Here's how the part is built. I have some questions about the finished solid (model axes, mm). Face numbers are marked on the shaded views. A direction names the side the tool comes from. Round coordinates to 2 decimals unless told otherwise and drop trailing zeros. Loops run counter-clockwise (first coordinate to the right, second up) from the corner with the lowest first, then second, coordinate; pieces in that order, holes last. Notation, with made-up numbers: (69.25, 65.25) - (90.25, 65.25) arc R8 ccw to (90.25, 71.25) - close; hole circle Ø7 at (32, -1.75). An arc over 180 degrees is marked (long way). Answer as a JSON object with one key per item and string values. Group by question number.
1) Will these pins go through, and if not, where does the flat tip stop? P1, Ø16.5, axis at y = -9, z = 69, coming from the -X side; P2, Ø16.5, axis at y = 9, z = 68.5, coming from the +X side; P3, Ø3, axis at x = 8, y = -3.5, coming from the -Z side; P4, Ø4.5, axis at x = 51.5, z = 33.23, coming from the +Y side.
2) I want a section at C-C, the plane x = 44.5. Please give me the cut outline in (y, z), then the cut area to 3 significant figures.
3) I want a section at D-D, the plane z = -2.5. Please give me the cut outline in (x, y), then the cut area to 3 significant figures.
4) I want a section at A-A, the plane z = -43. Please give me the cut outline in (x, y).
5) I want a section at B-B, the plane y = 16. Please give me the cut outline in (x, z).
6) Which directions (+Z, -Z, +X, -X, +Y, -Y) give clear straight access to the entire face, cutting with the end or side of a thin tool? Please do the marked faces 1, 2 and 3.
7) If I drill on line 1 along X through (y, z) = (1.5, -43); line 2 along Z through (x, y) = (-50, 14); line 3 along X through (y, z) = (-14, -9), over which ranges is the centre line in solid material (lowest first)? Write a range as [from, to].
from build123d import *

# Parameters (mm, degrees)
BASE_MODEL_DEPTH         = 19
F_5_0_5_DIAMETER_HOLE1_D = 5


with BuildPart() as part:
    # Top → Base Model (new, symmetric)
    with BuildSketch(Plane(origin=(0, 0, 0), x_dir=(1, 0, 0), z_dir=(0, 1, 0))):
        with BuildLine():
            Line((-5.390272104, 50.397653109), (-58.548817366, -28.484658378))
            ThreePointArc((-58.548817366, -28.484658378), (-59.931398216, -32.157094268), (-59.517033361, -36.059224064))
            Line((-59.517033361, -36.059224064), (-51, -60.234834557))
            Line((-51, -60.234834557), (-51, -75.234834557))
            Line((-51, -75.234834557), (51, -75.234834557))
            Line((51, -75.234834557), (51, -60.234834557))
            Line((51, -60.234834557), (59.517033361, -36.059224064))
            ThreePointArc((59.517033361, -36.059224064), (59.931398216, -32.157094268), (58.548817366, -28.484658378))
            Line((58.548817366, -28.484658378), (5.390272104, 50.397653109))
            ThreePointArc((5.390272104, 50.397653109), (3.052771705, 52.503683101), (0, 53.265165443))
            ThreePointArc((0, 53.265165443), (-3.052771705, 52.503683101), (-5.390272104, 50.397653109))
        make_face()
    extrude(amount=BASE_MODEL_DEPTH, both=True)

    # Ø5.0 (5) Diameter Hole1 (through all)
    with Locations(Plane(origin=(0, 19, 0), x_dir=(1, 0, 0), z_dir=(0, 1, 0))):
        with Locations((-51.5, -33.234834557), (0, 43), (51.5, -33.234834557)):
            Hole(F_5_0_5_DIAMETER_HOLE1_D / 2)


solid = part.part
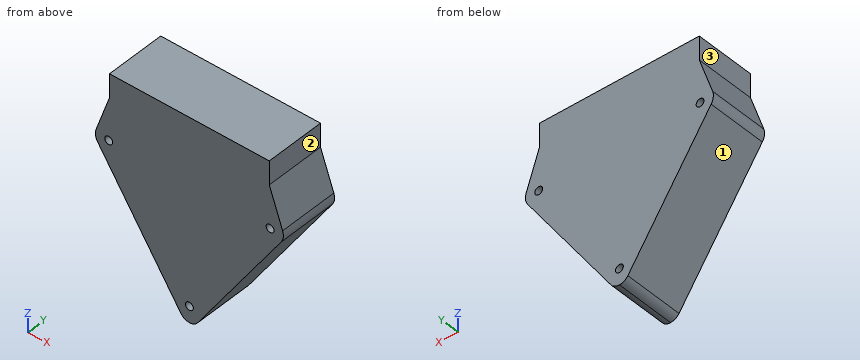
Outcome:
{
 "1": {"P1": "x = -51", "P2": "x = 51", "P3": "z = -48.75", "P4": "through"},
 "2": {"outline": "(-19, 7.64) - (19, 7.64) - (19, 75.23) - (-19, 75.23) - close", "area": "2,570 mm^2"},
 "3": {"outline": "(-37.67, -19) - (37.67, -19) - (37.67, 19) - (-37.67, 19) - close", "area": "2,860 mm^2"},
 "4": {"outline": "(-10.38, -19) - (-2.5, -19) - (-2.5, 19) - (-10.38, 19) - close; (2.5, -19) - (10.38, -19) - (10.38, 19) - (2.5, 19) - close"},
 "5": {"outline": "(-59.52, 36.06) arc R8.5 ccw to (-58.55, 28.48) - (-5.39, -50.4) arc R6.5 ccw to (5.39, -50.4) - (58.55, 28.48) arc R8.5 ccw to (59.52, 36.06) - (51, 60.23) - (51, 75.23) - (-51, 75.23) - (-51, 60.23) - close; hole circle Ø5 at (-51.5, 33.23); hole circle Ø5 at (0, -43); hole circle Ø5 at (51.5, 33.23)"},
 "6": {"face 1": "-Z, -X, +Y, -Y", "face 2": "+Z, +X, +Y, -Y", "face 3": "+Z, -X, +Y, -Y"},
 "7": {"line 1": "[-10.38, -2.5], [2.5, 10.38]", "line 2": "[15.8, 31.23], [35.23, 75.23]", "line 3": "[-33.29, 33.29]"}
}
